Design review of the part shown in the three views and the two pictorial views. Dimensions are in mm from the part's minimum x, y and z. Give positions to 0.01 mm unless a question says otherwise; leave off trailing zeros. Loops run counter-clockwise (first coordinate to the right, second up) from the corner with the lowest first, then second, coordinate; pieces in that order, holes last.
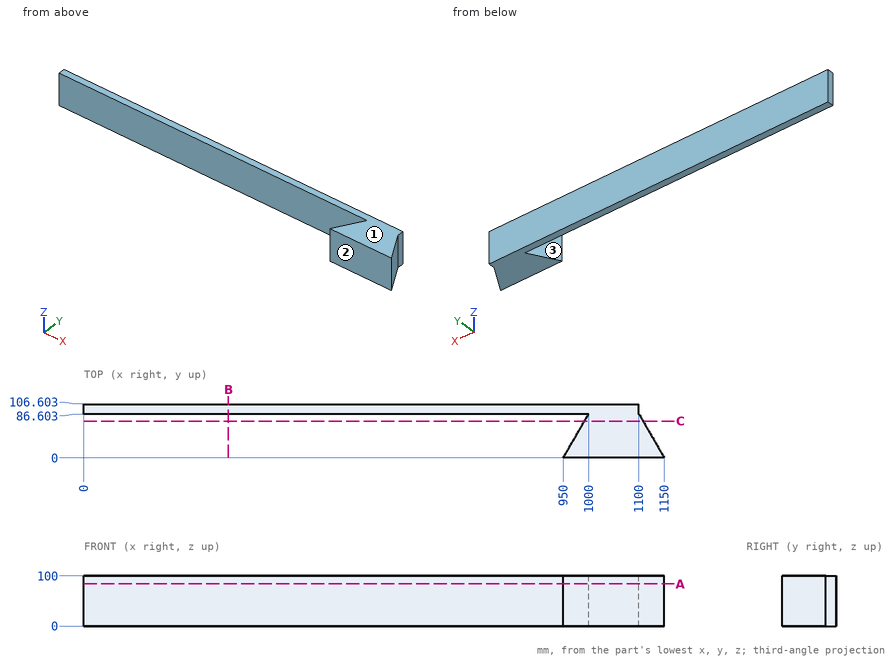
Q1. Draft analysis for pull direction Y (two halves, no side actions). For the marked faces 1, 2 and 3, state which applies: pulls with the +Y half, pulls with the -Y half, needs draft (parallel to the pull), parting line crosses it, or undercut.
Results:
face 1: needs draft
face 2: pulls with the -Y half
face 3: undercut
Q2. Wall thickness on line 1 (Y direction, x = 703, z = 36.5); line 2 (X direction, y = 12.5, z = 9.5) (1 decimal); line 3 (X direction, y = 78, z = 41.5) (1 decimal): over which ranges is each line inside the solid? List them lowest first.
Results:
line 1: y = 86.6 to 106.6
line 2: x = 957.2 to 1142.8
line 3: x = 995 to 1105
Q3. Take a section at B-B (x = 286). Give the boundary of the cut face in (y, z), plus the area to 3 significant figures.
Results:
outline: (86.6, 0) - (106.6, 0) - (106.6, 100) - (86.6, 100) - close
area: 2,000 mm2
Q4. Take a section at C-C (y = 72.5). Give the boundary of the cut face in (x, z), plus the area to 3 significant figures.
Results:
outline: (991.86, 0) - (1108.14, 0) - (1108.14, 100) - (991.86, 100) - close
area: 11,600 mm2
Q5. Take a section at A-A (z = 84). Give the boundary of the cut face in (x, y), plus the area to 3 significant figures.
Results:
outline: (0, 86.6) - (1000, 86.6) - (950, 0) - (1150, 0) - (1100, 86.6) - (1100, 106.6) - (0, 106.6) - close
area: 35,000 mm2
Q6. Insertion check: pin 1 (10 mm diameter, centred on x = 335.5, z = 45, fed in from -Y); pin 2 (10 mm diameter, centred on y = 49.5, z = 13.5, fed in from +X); pin 3 (10 mm diameter, centred on y = 97, z = 51, fed in from +X). Each pin has a flat end and moves straight along its axis. Give the tip position at first contact, or say it passes through.
Results:
pin 1: stops at y = 86.6
pin 2: stops at x = 1124.31
pin 3: stops at x = 1100
